Input: part model. Units: mm. Frame: model coordinates. A direction names the side the tool comes from. Coordinates: 2 decimals unless noted, no trailing zeros. Write each loop counter-clockwise with the first axis right and the second up, starting at its lowest first coordinate (ties: lowest second). Pieces come first, ordered by that corner, then holes.
1) Set-up query: faces 4 (the flat face through (6.8, 0, 2)), 5 (the flat face through (-6.8, 0, 2)), 6 (the flat face through (-1.4, -1.7, 1)). Return all of +Z, -Z, +X, -X, +Y, -Y with unobstructed straight access to the full face (end or side cutting, diameter ignored); none if empty.
2) Draft query along Y for faces 1 (the flat face through (0, 2.3, 3)), 2 (the cylindrical face through (-1.5, 0.07, 0.25)), 3 (the flat face through (0, 2.8, 2)). Return one class per face: pulls with the +Y half, pulls with the -Y half, needs draft (parallel to the pull), parting line crosses it, or undercut.
3) Pin query (flat end, axial travel): pin 1 Ø4 at (x, y) = (3.5, 0) entering from -Z; pin 2 Ø1 at (y, z) = (0, 2) entering from +X; pin 3 Ø1 at (y, z) = (-0.5, 2) entering from -X; pin 4 Ø0.6 at (x, z) = (1.5, 2) entering from +Y. Return the tip coordinate at first contact, or that it passes through.
4) Line query: L1, parallel to Y at x = 0, z = 0.15; L2, parallel to X at y = 0.25, z = 1.6; L3, parallel to Y at x = 2.75, z = 1.4. Output: solid intervals per line, ascending.
5) Section query A-A (y = 0). Output: boundary loops of the cut face in (x, z).
6) Section query D-D (y = 2.5). Output: boundary loops of the cut face in (x, z), then the cut area to 3 significant figures.
7) Section query C-C (z = 1.45). Output: boundary loops of the cut face in (x, y), then the cut area to 3 significant figures.
from build123d import *

# Parameters (mm, degrees)
F0_W     = 13.6
F0_H     = 5.6
F1_DEPTH = 3
F2_T     = -0.8
F3_W     = 16
F3_H     = 8
F4_DEPTH = 1
F5_R     = 0.75
F6_R     = 1
F7_R     = 1.5
F8_DEPTH = 25
F10_R    = 0.49999


# Not quite as in the source:
# - a fillet or chamfer is up to 0.001 mm smaller than in the source, because OpenCascade refuses the exact size


with BuildPart() as f1:
    # F0 (on Top) → F1 (new body)
    with BuildSketch(Plane.XY):
        Rectangle(F0_W, F0_H)
    extrude(amount=F1_DEPTH)

    # F2
    f2_openings = [f1.faces().sort_by_distance(p)[0] for p in [
        (0, 0, 3),
    ]]
    offset(amount=F2_T, openings=f2_openings)

    # F3 (on Top) → F4 (join)
    with BuildSketch(Plane.XY):
        Rectangle(F3_W, F3_H)
    extrude(amount=F4_DEPTH)

    # F5
    f5_edges = [f1.edges().sort_by_distance(p)[0] for p in [
        (6.8, -2.8, 2),
        (6.8, 2.8, 2),
        (6, 2, 2),
        (6, -2, 2),
        (-6, 2, 2),
        (-6, -2, 2),
        (-6.8, 2.8, 2),
        (-6.8, -2.8, 2),
    ]]
    fillet(f5_edges, radius=F5_R)

    # F6
    f6_edges = [f1.edges().sort_by_distance(p)[0] for p in [
        (-8, -4, 0.5),
        (8, -4, 0.5),
        (8, 4, 0.5),
        (-8, 4, 0.5),
    ]]
    fillet(f6_edges, radius=F6_R)


with BuildPart() as f8:
    # F7 (on Top) → F8 (new body)
    with BuildSketch(Plane.XY):
        Circle(F7_R)
    extrude(amount=F8_DEPTH)


with BuildPart() as f1_1:
    add(f1.part)

    # F9: cut F8
    add(f8.part, mode=Mode.SUBTRACT)

    # F10 (radius 0.5 in the source; OpenCascade refuses exactly that, so slightly less here)
    f10_edges = [f1_1.edges().sort_by_distance(p)[0] for p in [
        (-1.5, 0, 1),
    ]]
    fillet(f10_edges, radius=F10_R)


solid = f1_1.part
Answer:
1. face 4: +Z, +X, +Y, -Y
1. face 5: +Z, -X, +Y, -Y
1. face 6: +Z
2. face 1: needs draft
2. face 2: undercut
2. face 3: pulls with the +Y half
3. pin 1: stops at z = 0
3. pin 2: stops at x = 6.8
3. pin 3: stops at x = -6.8
3. pin 4: stops at y = 2.8
4. L1: y = -4 to -1.5, 1.5 to 4
4. L2: x = -6.8 to -6, 6 to 6.8
4. L3: y = -2.8 to -2, 2 to 2.8
5. outline: (-8, 0) - (-1.5, 0) - (-1.5, 0.5) arc R0.5 ccw to (-2, 1) - (-6, 1) - (-6, 3) - (-6.8, 3) - (-6.8, 1) - (-8, 1) - close; (1.5, 0) - (8, 0) - (8, 1) - (6.8, 1) - (6.8, 3) - (6, 3) - (6, 1) - (2, 1) arc R0.5 ccw to (1.5, 0.5) - close
6. outline: (-8, 0) - (8, 0) - (8, 1) - (6.65, 1) - (6.65, 3) - (-6.65, 3) - (-6.65, 1) - (-8, 1) - close
6. area: 42.6 mm2
7. outline: (-6.8, -2.05) arc R0.75 ccw to (-6.05, -2.8) - (6.05, -2.8) arc R0.75 ccw to (6.8, -2.05) - (6.8, 2.05) arc R0.75 ccw to (6.05, 2.8) - (-6.05, 2.8) arc R0.75 ccw to (-6.8, 2.05) - close; hole (-6, -1.25) arc R0.75 ccw to (-5.25, -2) - (5.25, -2) arc R0.75 ccw to (6, -1.25) - (6, 1.25) arc R0.75 ccw to (5.25, 2) - (-5.25, 2) arc R0.75 ccw to (-6, 1.25) - close
7. area: 28.2 mm2
